```python
from build123d import *

# Parameters (mm, degrees)
BOSS_EXTRUDE1_DEPTH = 4
CUT_EXTRUDE1_DEPTH  = 10


with BuildPart() as part:
    # Sketch1 → Boss-Extrude1 (new body)
    with BuildSketch(Plane(origin=(0, 0, 0), x_dir=(1, 0, 0), z_dir=(0, 1, 0))):
        Polygon((-17.714285714, -42), (-17.714285714, -32), (-21.714285714, -32), (-21.714285714, -28), (-17.714285714, -28), (-17.714285714, -16), (-21.714285714, -16), (-21.714285714, -12), (-17.714285714, -12), (-17.714285714, 0), (-21.714285714, 0), (-21.714285714, 4), (-17.714285714, 4), (-17.714285714, 14), (78.285714286, 14), (78.285714286, 4), (82.285714286, 4), (82.285714286, 0), (78.285714286, 0), (78.285714286, -12), (82.285714286, -12), (82.285714286, -16), (78.285714286, -16), (78.285714286, -28), (82.285714286, -28), (82.285714286, -32), (78.285714286, -32), (78.285714286, -42), align=None)
    extrude(amount=-BOSS_EXTRUDE1_DEPTH)

    # Sketch2 → Cut-Extrude1 (cut)
    with BuildSketch(Plane(origin=(0, 0, 0), x_dir=(1, 0, 0), z_dir=(0, 1, 0))):
        with BuildLine():
            Line((-2.595319649, 10), (25.285714286, 10))
            ThreePointArc((25.285714286, 10), (26.699927848, 9.414213562), (27.285714286, 8))
            Line((27.285714286, 8), (27.285714286, -4.273399853))
            ThreePointArc((27.285714286, -4.273399853), (26.378511973, -5.948450065), (24.479921071, -6.103890851))
            Line((24.479921071, -6.103890851), (-3.401112863, 6.169509001))
            ThreePointArc((-3.401112863, 6.169509001), (-4.552483668, 8.411714709), (-2.595319649, 10))
        make_face()
        with BuildLine():
            ThreePointArc((-13.714285714, 3.273399853), (-12.807083402, 4.948450065), (-10.9084925, 5.103890851))
            Line((-10.9084925, 5.103890851), (16.972541435, -7.169509001))
            ThreePointArc((16.972541435, -7.169509001), (18.12391224, -9.411714709), (16.16674822, -11))
            Line((16.16674822, -11), (-11.714285714, -11))
            ThreePointArc((-11.714285714, -11), (-13.128499277, -10.414213562), (-13.714285714, -9))
            Line((-13.714285714, -9), (-13.714285714, 3.273399853))
        make_face()
        with BuildLine():
            Line((33.285714286, 8), (33.285714286, -4.273399853))
            ThreePointArc((33.285714286, -4.273399853), (34.192916598, -5.948450065), (36.0915075, -6.103890851))
            Line((36.0915075, -6.103890851), (63.972541435, 6.169509001))
            ThreePointArc((63.972541435, 6.169509001), (65.12391224, 8.411714709), (63.16674822, 10))
            Line((63.16674822, 10), (35.285714286, 10))
            ThreePointArc((35.285714286, 10), (33.871500723, 9.414213562), (33.285714286, 8))
        make_face()
        with BuildLine():
            ThreePointArc((74.285714286, -9), (73.699927848, -10.414213562), (72.285714286, -11))
            Line((72.285714286, -11), (44.404680351, -11))
            ThreePointArc((44.404680351, -11), (42.447516332, -9.411714709), (43.598887137, -7.169509001))
            Line((43.598887137, -7.169509001), (71.479921071, 5.103890851))
            ThreePointArc((71.479921071, 5.103890851), (73.378511973, 4.948450065), (74.285714286, 3.273399853))
            Line((74.285714286, 3.273399853), (74.285714286, -9))
        make_face()
        with BuildLine():
            ThreePointArc((74.285714286, -31.273399853), (73.378511973, -32.948450065), (71.479921071, -33.103890851))
            Line((71.479921071, -33.103890851), (43.598887137, -20.830490999))
            ThreePointArc((43.598887137, -20.830490999), (42.447516332, -18.588285291), (44.404680351, -17))
            Line((44.404680351, -17), (72.285714286, -17))
            ThreePointArc((72.285714286, -17), (73.699927848, -17.585786438), (74.285714286, -19))
            Line((74.285714286, -19), (74.285714286, -31.273399853))
        make_face()
        with BuildLine():
            Line((63.16674822, -38), (35.285714286, -38))
            ThreePointArc((35.285714286, -38), (33.871500723, -37.414213562), (33.285714286, -36))
            Line((33.285714286, -36), (33.285714286, -23.726600147))
            ThreePointArc((33.285714286, -23.726600147), (34.192916598, -22.051549935), (36.0915075, -21.896109149))
            Line((36.0915075, -21.896109149), (63.972541435, -34.169509001))
            ThreePointArc((63.972541435, -34.169509001), (65.12391224, -36.411714709), (63.16674822, -38))
        make_face()
        with BuildLine():
            Line((27.285714286, -36), (27.285714286, -23.726600147))
            ThreePointArc((27.285714286, -23.726600147), (26.378511973, -22.051549935), (24.479921071, -21.896109149))
            Line((24.479921071, -21.896109149), (-3.401112863, -34.169509001))
            ThreePointArc((-3.401112863, -34.169509001), (-4.552483668, -36.411714709), (-2.595319649, -38))
            Line((-2.595319649, -38), (25.285714286, -38))
            ThreePointArc((25.285714286, -38), (26.699927848, -37.414213562), (27.285714286, -36))
        make_face()
        with BuildLine():
            ThreePointArc((-13.714285714, -19), (-13.128499277, -17.585786438), (-11.714285714, -17))
            Line((-11.714285714, -17), (16.16674822, -17))
            ThreePointArc((16.16674822, -17), (18.12391224, -18.588285291), (16.972541435, -20.830490999))
            Line((16.972541435, -20.830490999), (-10.9084925, -33.103890851))
            ThreePointArc((-10.9084925, -33.103890851), (-12.807083402, -32.948450065), (-13.714285714, -31.273399853))
            Line((-13.714285714, -31.273399853), (-13.714285714, -19))
        make_face()
    extrude(amount=-CUT_EXTRUDE1_DEPTH, mode=Mode.SUBTRACT)


solid = part.part
```
Read the model definition and answer for the solid it produces. Units are mm, in the model's axes. A direction names the side the tool comes from. Coordinates: 2 decimals unless noted, no trailing zeros. Loops run counter-clockwise (first coordinate to the right, second up) from the corner with the lowest first, then second, coordinate; pieces in that order, holes last. Notation, with made-up numbers: (89.5, -22) -> (97.5, -22) arc R13 ccw to (97.5, -14) -> close; hole circle Ø10 at (47, 21.25). An arc over 180 degrees is marked (long way). Return JSON: item names as keys, results as strings.
Item 1: For a pull along X with two mould halves and no side action, classify faces 1 (the flat face through (78.286, -2, -9)), 2 (the flat face through (74.286, -2, 3)), 3 (the flat face through (31, 0, 14)) as +X half, -X half, draft (parallel to the pull), parting line (faces both ways), or undercut.
Answers:
{"face 1": "+X half", "face 2": "undercut", "face 3": "draft"}
Item 2: Find section A-A (x = 4). Determine the outline of the cut face in (y, z).
Answers:
{"outline": "(-4, -14) -> (0, -14) -> (0, -10) -> (-4, -10) -> close; (-4, -2.91) -> (0, -2.91) -> (0, 1.46) -> (-4, 1.46) -> close; (-4, 11) -> (0, 11) -> (0, 17) -> (-4, 17) -> close; (-4, 26.54) -> (0, 26.54) -> (0, 30.91) -> (-4, 30.91) -> close; (-4, 38) -> (0, 38) -> (0, 42) -> (-4, 42) -> close"}
Item 3: Find the intervals of material crossed by probe 1 along X at (y, z) = (-0.35, -8); probe 2 along Z at (x, y) = (17.5, -0.6); probe 3 along Z at (x, y) = (4, -3.5), in increasing order.
Answers:
{"probe 1": "x = -17.71 to -4.6, 27.29 to 33.29, 65.17 to 78.29", "probe 2": "z = -14 to -10, 3.03 to 7.51, 10.49 to 17.51, 20.49 to 24.97, 38 to 42", "probe 3": "z = -14 to -10, -2.91 to 1.46, 11 to 17, 26.54 to 30.91, 38 to 42"}
Item 4: Find section B-B (y = -1). Count the separate pieces of the cut face and the enclosed holes in it, plus the area to 3 significant figures.
Answers:
{"separate pieces": "1", "enclosed holes": "8", "area": "2,870 mm2"}
Item 5: Flat-ended cylindrical pins translate along their axes: P1, Ø1.2, axis at x = -19.5, y = -2.5, coming from the -Z side; P2, Ø1.2, axis at y = -2.5, z = 32.5, coming from the -X side; P3, Ø2, axis at x = -19, y = -3, coming from the +Z side; P4, Ø1.2, axis at y = -2.5, z = 4, coming from the +X side. Find the tip coordinate at first contact, or state that the pin passes through.
Answers:
{"P1": "stops at z = -4", "P2": "stops at x = -21.71", "P3": "stops at z = 32", "P4": "stops at x = 78.29"}
Item 6: For faces 4 (the cylindrical face through (33.89, -1.97, 37.43)), 5 (the flat face through (-20, -2, 28)), determine the directions among +Z, -Z, +X, -X, +Y, -Y from which every point of the face is accessible in a straight line to the end or side of a thin tool.
Answers:
{"face 4": "+Y, -Y", "face 5": "-X, +Y, -Y"}
